Could you check a few things on this drawing? It's one solid part, dimensions in mm from its lowest x, y, z. A direction names the side the tool comes from. Coordinates: 2 decimals unless noted, no trailing zeros. Order: outer loops, then holes, each group sorted by start corner. A loop starts at its lowest first (then second) coordinate and runs counter-clockwise, first axis right, second up. Notation, with made-up numbers: (23, 65) -> (27, 65) arc R24 ccw to (27, 78) -> close; hole circle Ø11 at (6.5, 43.25). An arc over 180 degrees is marked (long way). Answer as CSV lines item,"result".
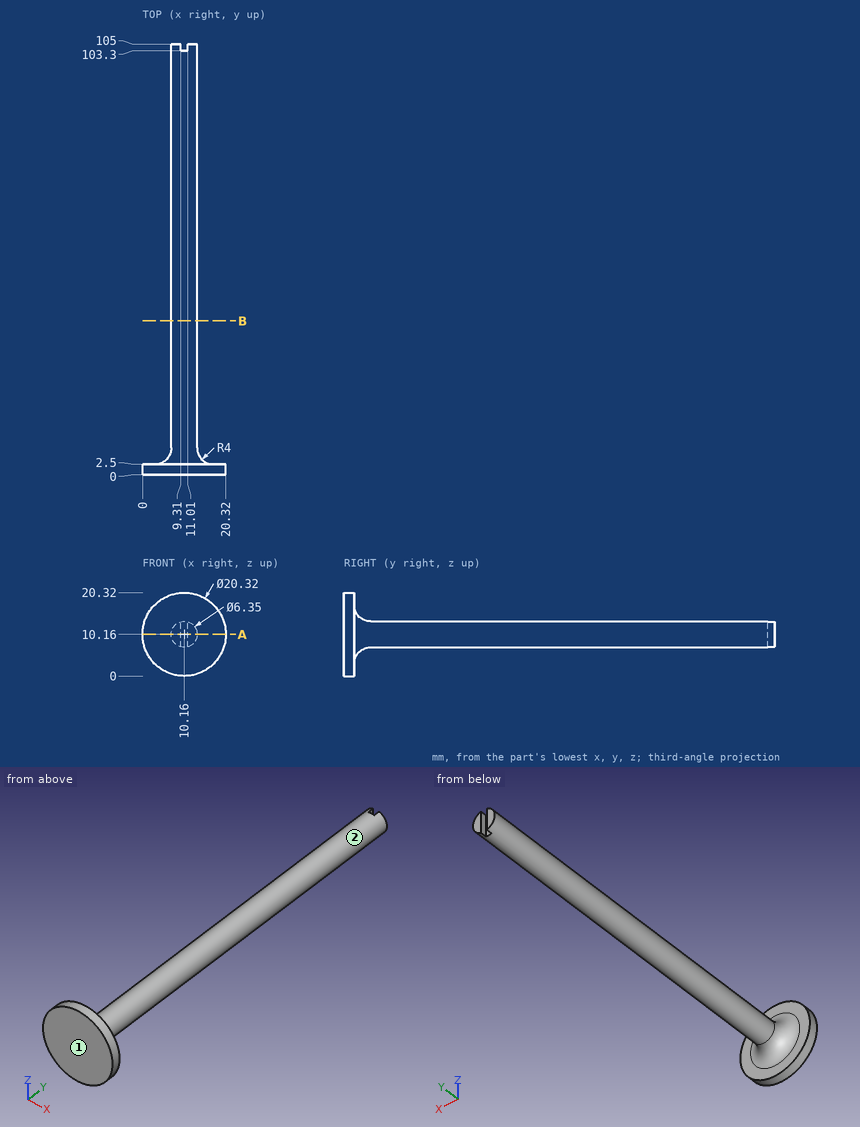
Q1. If I drill on line 1 (X direction, y = 82, z = 10.5); line 2 (Z direction, x = 10, y = 24.5); line 3 (X direction, y = 37.5, z = 11), over which ranges is the centre line in solid material (lowest first)?
Solution:
line 1,"7 to 13.32"
line 2,"6.99 to 13.33"
line 3,"7.1 to 13.22"
Q2. Which directions (+Z, -Z, +X, -X, +Y, -Y) give clear straight access to the entire face, cutting with the end or side of a thin tool? Please do the marked faces 1 and 2.
Solution:
face 1,"+Z, -Z, +X, -X, -Y"
face 2,"+Y"
Q3. For P1, Ø12, axis at y = 34.5, z = 3.5, coming from the -X side; P2, Ø10, axis at x = 9, y = 16.5, coming from the +Z side (3 decimals); P3, Ø3, axis at y = 32, z = 7.5, coming from the -X side, each with a flat end and sliding along its axis, tell me the tip position at first contact or that it passes through.
Solution:
P1,"x = 7.05"
P2,"z = 13.335"
P3,"x = 7.2"
Q4. Imagine slicing it at A-A (z = 10.16). List the corners of the cut face in (x, y) for me (3 decimals), and give its area (3 significant figures).
Solution:
outline,"(0, 0) -> (20.32, 0) -> (20.32, 2.5) -> (17.335, 2.5) arc R4 cw to (13.335, 6.5) -> (13.335, 105) -> (11.01, 105) -> (11.01, 103.3) -> (9.31, 103.3) -> (9.31, 105) -> (6.985, 105) -> (6.985, 6.5) arc R4 cw to (2.985, 2.5) -> (0, 2.5) -> close"
area,"706 mm2"
Q5. Imagine slicing it at B-B (y = 37.5). List the corners of the cut face in (x, z) for me (3 decimals), and give its area (3 significant figures).
Solution:
outline,"circle Ø6.35 at (10.16, 10.16)"
area,"31.7 mm2"
